from build123d import *

# Parameters (mm, degrees)
BOSS_EXTRUDE4_DEPTH           = 25
CUT_EXTRUDE2_DEPTH            = 25
TAP_DRILL_FOR_4_40_TAP1_D     = 1.600000102
TAP_DRILL_FOR_4_40_TAP1_DEPTH = 7.874
TAP_DRILL_FOR_4_40_TAP1_TIP   = 0.480688526
TAP_DRILL_FOR_4_40_TAP3_D     = 1.600000102
TAP_DRILL_FOR_4_40_TAP3_DEPTH = 7.874
TAP_DRILL_FOR_4_40_TAP3_TIP   = 0.480688526
TAP_DRILL_FOR_4_40_TAP4_D     = 1.600000102
TAP_DRILL_FOR_4_40_TAP4_DEPTH = 7.874
TAP_DRILL_FOR_4_40_TAP4_TIP   = 0.480688526
FILLET1_R                     = 1.778
CUT_EXTRUDE3_DEPTH            = 2.5
CUT_EXTRUDE4_DEPTH            = 2.5
CUT_EXTRUDE5_DEPTH            = 2.5
SKETCH23_W                    = 11
SKETCH23_H                    = 5.045
CUT_EXTRUDE6_DEPTH            = 5
SKETCH24_W                    = 11
SKETCH24_H                    = 5.045
CUT_EXTRUDE7_DEPTH            = 5
SKETCH25_W                    = 11
SKETCH25_H                    = 16.07506189
CUT_EXTRUDE8_DEPTH            = 10
SKETCH26_W                    = 184.458934752
SKETCH26_H                    = 50.4
BOSS_EXTRUDE6_DEPTH           = 29.21
SKETCH27_R                    = 3.429
CUT_EXTRUDE9_DEPTH            = 106.37252383


with BuildPart() as part:
    # Sketch6 → Boss-Extrude4 (new body)
    with BuildSketch(Plane(origin=(0, 0, 0), x_dir=(1, 0, 0), z_dir=(0, 1, 0))):
        Polygon((-79.529467376, 0), (79.529467376, 0), (79.529467376, -56.321059428), (25, -63.5), (-25, -63.5), (-79.529467376, -56.321059428), align=None)
    extrude(amount=BOSS_EXTRUDE4_DEPTH)

    # Sketch7 → Cut-Extrude2 (cut, symmetric)
    with BuildSketch(Plane(origin=(0, 0, 0), x_dir=(0, 0, -1), z_dir=(1, 0, 0))):
        Polygon((-63.5, 25), (-38.5, 0), (-63.5, 0), align=None)
    extrude(amount=CUT_EXTRUDE2_DEPTH, both=True, mode=Mode.SUBTRACT)

    # Tap Drill for #4-40 Tap1
    with Locations(Plane(origin=(0, -19.25, 19.25), x_dir=(-1, 0, 0), z_dir=(0, -0.7071067811865488, 0.7071067811865462))):
        with Locations((-21.255000035, -53.756280605), (21.255000035, -53.756280605), (21.255000035, -36.046280605), (-21.255000035, -36.046280605)):
            Hole(TAP_DRILL_FOR_4_40_TAP1_D / 2, depth=TAP_DRILL_FOR_4_40_TAP1_DEPTH)
            with Locations((0, 0, -(TAP_DRILL_FOR_4_40_TAP1_DEPTH + TAP_DRILL_FOR_4_40_TAP1_TIP / 2))):  # 118° drill point
                Cone(0, TAP_DRILL_FOR_4_40_TAP1_D / 2, TAP_DRILL_FOR_4_40_TAP1_TIP, mode=Mode.SUBTRACT)

    # Tap Drill for #4-40 Tap3
    with Locations(Plane(origin=(-8.643431853, 0, 65.653383048), x_dir=(0.9914448613738104, 0, 0.13052619222005213), z_dir=(-0.13052619222005213, 0, 0.9914448613738104))):
        with Locations((-65.252708328, 21.355), (-22.742708328, 21.355), (-22.742708328, 3.645), (-65.252708328, 3.645)):
            Hole(TAP_DRILL_FOR_4_40_TAP3_D / 2, depth=TAP_DRILL_FOR_4_40_TAP3_DEPTH)
            with Locations((0, 0, -(TAP_DRILL_FOR_4_40_TAP3_DEPTH + TAP_DRILL_FOR_4_40_TAP3_TIP / 2))):  # 118° drill point
                Cone(0, TAP_DRILL_FOR_4_40_TAP3_D / 2, TAP_DRILL_FOR_4_40_TAP3_TIP, mode=Mode.SUBTRACT)

    # Tap Drill for #4-40 Tap4
    with Locations(Plane(origin=(8.643431853, 0, 65.653383048), x_dir=(0.9914448613738104, 0, -0.13052619222005213), z_dir=(0.13052619222005213, 0, 0.9914448613738104))):
        with Locations((22.742708328, 21.355), (65.252708328, 21.355), (65.252708328, 3.645), (22.742708328, 3.645)):
            Hole(TAP_DRILL_FOR_4_40_TAP4_D / 2, depth=TAP_DRILL_FOR_4_40_TAP4_DEPTH)
            with Locations((0, 0, -(TAP_DRILL_FOR_4_40_TAP4_DEPTH + TAP_DRILL_FOR_4_40_TAP4_TIP / 2))):  # 118° drill point
                Cone(0, TAP_DRILL_FOR_4_40_TAP4_D / 2, TAP_DRILL_FOR_4_40_TAP4_TIP, mode=Mode.SUBTRACT)

    # Fillet1
    fillet1_edges = [part.edges().sort_by_distance(p)[0] for p in [
        (-79.529467376, 25, 28.160529714),
        (79.529467376, 25, 28.160529714),
        (-79.529467376, 0, 28.160529714),
        (79.529467376, 0, 28.160529714),
    ]]
    fillet(fillet1_edges, radius=FILLET1_R)

    # Sketch22 → Cut-Extrude3 (cut)
    with BuildSketch(Plane(origin=(0, -19.25, 19.25), x_dir=(1, 0, 0), z_dir=(0, -0.7071067811865488, 0.7071067811865462))):
        Polygon((-19.055000086, 53.756280605), (-19.055000086, 50.756280605), (-22.055000086, 50.756280605), (-22.055000086, 39.046280605), (-19.055000086, 39.046280605), (-19.055000086, 36.046280605), (19.055000086, 36.046280605), (19.055000086, 39.046280605), (22.055000086, 39.046280605), (22.055000086, 50.756280605), (19.055000086, 50.756280605), (19.055000086, 53.756280605), align=None)
    extrude(amount=-CUT_EXTRUDE3_DEPTH, mode=Mode.SUBTRACT)

    # Sketch21 → Cut-Extrude4 (cut)
    with BuildSketch(Plane(origin=(8.643431853, 0, 65.653383048), x_dir=(0.9914448613738104, 0, -0.13052619222005213), z_dir=(0.13052619222005213, 0, 0.9914448613738104))):
        Polygon((24.942708277, 21.355), (24.942708277, 18.355), (21.942708277, 18.355), (21.942708277, 6.645), (24.942708277, 6.645), (24.942708277, 3.645), (63.052708379, 3.645), (63.052708379, 6.645), (66.052708379, 6.645), (66.052708379, 18.355), (63.052708379, 18.355), (63.052708379, 21.355), align=None)
    extrude(amount=-CUT_EXTRUDE4_DEPTH, mode=Mode.SUBTRACT)

    # Sketch20 → Cut-Extrude5 (cut)
    with BuildSketch(Plane(origin=(-8.643431853, 0, 65.653383048), x_dir=(0.9914448613738104, 0, 0.13052619222005213), z_dir=(-0.13052619222005213, 0, 0.9914448613738104))):
        Polygon((-63.052708379, 21.355), (-63.052708379, 18.355), (-66.052708379, 18.355), (-66.052708379, 6.645), (-63.052708379, 6.645), (-63.052708379, 3.645), (-24.942708277, 3.645), (-24.942708277, 6.645), (-21.942708277, 6.645), (-21.942708277, 18.355), (-24.942708277, 18.355), (-24.942708277, 21.355), align=None)
    extrude(amount=-CUT_EXTRUDE5_DEPTH, mode=Mode.SUBTRACT)

    # Sketch23 → Cut-Extrude6 (cut)
    with BuildSketch(Plane(origin=(8.643431853, 0, 65.653383048), x_dir=(0.9914448613738104, 0, -0.13052619222005213), z_dir=(0.13052619222005213, 0, 0.9914448613738104))):
        with Locations((43.997708328, 2.5225)):
            Rectangle(SKETCH23_W, SKETCH23_H)
    extrude(amount=-CUT_EXTRUDE6_DEPTH, mode=Mode.SUBTRACT)

    # Sketch24 → Cut-Extrude7 (cut)
    with BuildSketch(Plane(origin=(-8.643431853, 0, 65.653383048), x_dir=(0.9914448613738104, 0, 0.13052619222005213), z_dir=(-0.13052619222005213, 0, 0.9914448613738104))):
        with Locations((-43.997708328, 2.5225)):
            Rectangle(SKETCH24_W, SKETCH24_H)
    extrude(amount=-CUT_EXTRUDE7_DEPTH, mode=Mode.SUBTRACT)

    # Sketch25 → Cut-Extrude8 (cut)
    with BuildSketch(Plane(origin=(0, -19.25, 19.25), x_dir=(1, 0, 0), z_dir=(0, -0.7071067811865488, 0.7071067811865462))):
        with Locations((0, 29.40874966)):
            Rectangle(SKETCH25_W, SKETCH25_H)
    extrude(amount=-CUT_EXTRUDE8_DEPTH, mode=Mode.SUBTRACT)

    # Sketch26 → Boss-Extrude6 (add)
    with BuildSketch(Plane(origin=(0, 0, 0), x_dir=(-1, 0, 0), z_dir=(0, 0, -1))):
        with Locations((0, 12.5)):
            Rectangle(SKETCH26_W, SKETCH26_H)
    extrude(amount=-BOSS_EXTRUDE6_DEPTH)

    # Sketch11 → Cut-Revolve4 (revolve, cut)
    with BuildSketch(Plane(origin=(0, 0, 0), x_dir=(0, 0, -1), z_dir=(1, 0, 0))):
        with BuildLine():
            Line((1344.295, -496.77), (1344.295, 521.77))
            add(Edge.make_bspline(
                [(1344.295, 521.77), (-28.575, 521.77), (-28.575, 12.5), (-28.575, -496.77), (1344.295, -496.77)],
                knots=[4.71238898, 4.71238898, 4.71238898, 6.283185307, 6.283185307, 7.853981634, 7.853981634, 7.853981634], degree=2, weights=[1, 0.707106781, 1, 0.707106781, 1]))
        make_face()
    revolve(axis=Axis((0, -496.77, -1344.295), (0, 1, 0)), mode=Mode.SUBTRACT)

    # Sketch27 → Cut-Extrude9 (cut, through all)
    with BuildSketch(Plane.XY.offset(29.21)):
        with Locations((85.879467376, -6.35)):
            Circle(SKETCH27_R)
        with Locations((-85.879467376, -6.35)):
            Circle(SKETCH27_R)
        with Locations((-85.879467376, 31.35)):
            Circle(SKETCH27_R)
        with Locations((85.879467376, 31.35)):
            Circle(SKETCH27_R)
    extrude(amount=-CUT_EXTRUDE9_DEPTH, mode=Mode.SUBTRACT)


solid = part.part
Build history of the part. All positions in model axes, mm. A direction names the side the tool comes from. Round coordinates to 2 decimals unless told otherwise and drop trailing zeros. Write each loop counter-clockwise with the first axis right and the second up, starting at its lowest first coordinate (ties: lowest second). Pieces come first, ordered by that corner, then holes. Notation, with made-up numbers: (-23, -9) - (-11, -9) arc R23 cw to (-11, 11) - close; hole circle Ø1 at (20.25, -10). An arc over 180 degrees is marked (long way). Use CSV: the item, a comma, the result in double quotes.
(1) Pin check, flat tips, straight feed: P1, Ø15.5, axis at y = 7.5, z = 36, coming from the +X side; P2, Ø7.5, axis at y = 16.5, z = 50, coming from the -X side; P3, Ø2, axis at x = 44.5, z = 58.5, coming from the -Y side; P4, Ø6, axis at x = -4.5, y = 25, coming from the +Z side. Stop position of each tip, or through.
Response:
P1,"x = 92.23"
P2,"x = -79.53"
P3,"y = 0"
P4,"z = 63.5"
(2) Mould opens along Y. For faces 1 (the flat face through (25, 7, 56)), 2 (the cylindrical face through (-20.492, 21.414, 54.269)), 3 (the flat face through (0.4, 21, 59.5)) say: pulls with the +Y half, pulls with the -Y half, needs draft (parallel to the pull), parting line crosses it, or undercut.
Response:
face 1,"needs draft"
face 2,"undercut"
face 3,"pulls with the -Y half"
(3) Band-saw the part on A-A (z = 35.5). Write the cut outline in (x, y).
Response:
outline,"(-79.53, 1.78) arc R1.78 ccw to (-77.75, 0) - (-5.5, 0) - (-5.5, 11.14) - (5.5, 11.14) - (5.5, 0) - (77.75, 0) arc R1.78 ccw to (79.53, 1.78) - (79.53, 23.22) arc R1.78 ccw to (77.75, 25) - (-77.75, 25) arc R1.78 ccw to (-79.53, 23.22) - close"
(4) Wall check: line 1 (Y direction, x = -59, z = 57) (3 decimals); line 2 (X direction, y = 7.5, z = 48.5); line 3 (Y direction, x = 61, z = 38). Give the ranges that are in metal, low to high.
Response:
line 1,"0 to 3.645, 21.355 to 25"
line 2,"-79.53 to -25, 25 to 79.53"
line 3,"0 to 25"
(5) 3-axis set-ups, long thin cutter, end or side, ignore diameter. For faces 4 (the flat face through (1, -12.7, 28)), 5 (the flat face through (-79.529, 12, 43)), 6 (the flat face through (52, 21.355, 59)), 7 (the flat face through (18, 0, 38)), 8 (the flat face through (1, 25, 46)): which of +Z, -Z, +X, -X, +Y, -Y reach the whole face in a straight line?
Response:
face 4,"+Z, -Z, +X, -X, -Y"
face 5,"+Z, -X, +Y, -Y"
face 6,"+Z"
face 7,"+Z, +X, -X, -Y"
face 8,"+Z, +X, -X, +Y"
